The listing builds one solid part. Answer for the finished solid, in the listing's coordinates (mm). Face numbers are marked on the shaded views. Give positions to 0.01 mm unless a question says otherwise; leave off trailing zeros. Loops run counter-clockwise (first coordinate to the right, second up) from the corner with the lowest first, then second, coordinate; pieces in that order, holes last. Notation, with made-up numbers: (50.25, -10.5) - (60.25, -10.5) arc R35 cw to (60.25, 28.5) - close; hole circle Ø2 at (53.25, -11.5). An arc over 180 degrees is marked (long way). Write item = value, one per line. Start each with the question number.
1) The part is cut by section A-A on y = 0. Write down the section's boundary in (x, z).
2) Consider probe 1 along X at (y, z) = (-1.3, 0.9); probe 2 along X at (y, z) = (-0.1, 0.5); probe 3 along Y at (x, z) = (11, 0.35). Determine where each line is inside the solid, lowest interval first.
3) The part is cut by section C-C on x = -0.25. Write down the section's boundary in (y, z), plus the area to 3 significant figures.
4) The mould has two halves that part along X. Classify the marked faces 1, 2 and 3: +X half, -X half, draft (parallel to the pull), parting line (faces both ways), or undercut.
5) Flat-ended cylindrical pins translate along their axes: P1, Ø1.5, axis at x = 9, z = -0.5, coming from the -Y side; P2, Ø1.5, axis at x = 0.5, z = 0, coming from the +Y side; P3, Ø2, axis at x = 10, z = -1.5, coming from the -Y side. Find the tip coordinate at first contact, or state that the pin passes through.
6) The part is cut by section B-B on x = 1.5. Write down the section's boundary in (y, z), plus the area to 3 significant figures.
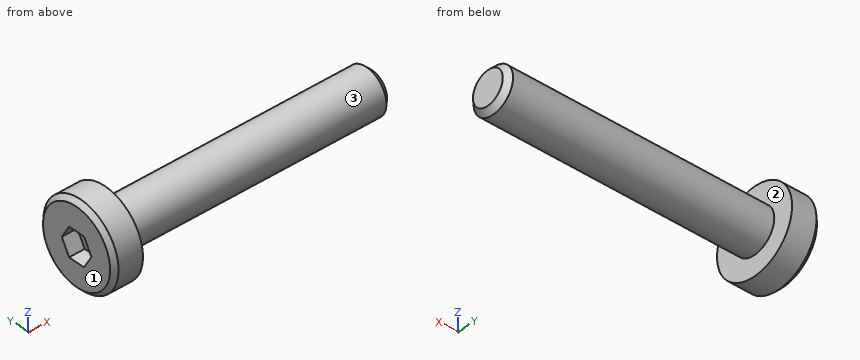
from build123d import *

# Parameters (mm, degrees)
CUT_EXTRUDE1_DEPTH = 0.7


with BuildPart() as part:
    # Sketch1 → Revolve1 (revolve)
    with BuildSketch(Plane.XY):
        Polygon((-1.3, 0), (-1.3, 1.7), (-1.1, 1.9), (0, 1.9), (0, 1), (11.7545, 1), (12, 0.7545), (12, 0), align=None)
    revolve(axis=Axis((12, 0, 0), (-1, 0, 0)))

    # Sketch2 → Cut-Extrude1 (cut)
    with BuildSketch(Plane(origin=(-1.3, 0, 0), x_dir=(0, 0, -1), z_dir=(1, 0, 0))):
        Polygon((-0.65, -0.375277675), (0, -0.75055535), (0.65, -0.375277675), (0.65, 0.375277675), (0, 0.75055535), (-0.65, 0.375277675), align=None)
    extrude(amount=CUT_EXTRUDE1_DEPTH, mode=Mode.SUBTRACT)


solid = part.part
Answer below:
q1.outline = (-1.3, -1.7) - (-1.1, -1.9) - (0, -1.9) - (0, -1) - (11.75, -1) - (12, -0.75) - (12, 0.75) - (11.75, 1) - (0, 1) - (0, 1.9) - (-1.1, 1.9) - (-1.3, 1.7) - (-1.3, 0.65) - (-0.6, 0.65) - (-0.6, -0.65) - (-1.3, -0.65) - close
q2.probe_1 = -1.3 to 0
q2.probe_2 = -0.6 to 12
q2.probe_3 = -0.94 to 0.94
q3.outline = circle Ø3.8 at (0, 0)
q3.area = 11.3 mm2
q4.face_1 = -X half
q4.face_2 = +X half
q4.face_3 = draft
q5.P1 = -1
q5.P2 = 1.9
q5.P3 = -0.87
q6.outline = circle Ø2 at (0, 0)
q6.area = 3.14 mm2
